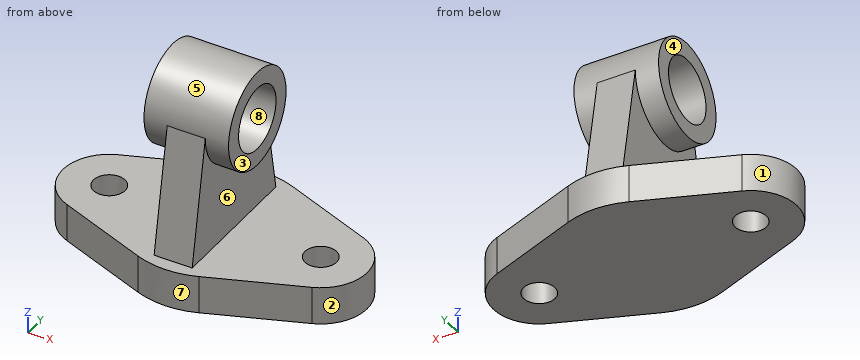
```python
from build123d import *

# Parameters (mm, degrees)
BOSS_EXTRUDE1_DEPTH = 18
SKETCH3_W           = 18
SKETCH3_H           = 67
BOSS_EXTRUDE2_DEPTH = 58
SKETCH4_R           = 23
BOSS_EXTRUDE3_DEPTH = 29
BOSS_EXTRUDE4_START = -40
SKETCH5_R           = 23
BOSS_EXTRUDE4_DEPTH = 40
SKETCH6_R           = 15
CUT_EXTRUDE1_DEPTH  = 141.943250991
CUT_EXTRUDE2_DEPTH  = 135.02238619
SKETCH8_R           = 7.5
CUT_EXTRUDE3_DEPTH  = 116.52056094


with BuildPart() as part:
    # Sketch2 → Boss-Extrude1 (new body)
    with BuildSketch(Plane.XY):
        with BuildLine():
            Line((-57.919997401, 20.524958004), (-14.399995275, 37.31809395))
            ThreePointArc((-14.399995275, 37.31809395), (0, 40), (14.399995275, 37.31809395))
            Line((14.399995275, 37.31809395), (57.919997401, 20.524958004))
            ThreePointArc((57.919997401, 20.524958004), (72, 9.117e-06), (57.920002599, -20.524943336))
            Line((57.920002599, -20.524943336), (14.399995275, -37.31809395))
            ThreePointArc((14.399995275, -37.31809395), (-5.065e-06, -40), (-14.400004725, -37.318090304))
            Line((-14.400004725, -37.318090304), (-57.920002599, -20.524943336))
            ThreePointArc((-57.920002599, -20.524943336), (-72, 9.117e-06), (-57.919997401, 20.524958004))
        make_face()
    extrude(amount=BOSS_EXTRUDE1_DEPTH)

    # Sketch3 → Boss-Extrude2 (add)
    with BuildSketch(Plane.XY.offset(18)):
        Rectangle(SKETCH3_W, SKETCH3_H)
    extrude(amount=BOSS_EXTRUDE2_DEPTH)

    # Sketch4 → Boss-Extrude3 (add)
    with BuildSketch(Plane(origin=(9, 0, 0), x_dir=(0, 0, -1), z_dir=(1, 0, 0))):
        with Locations(Location((-76, 0, 0), (0, 0, 90))):
            Circle(SKETCH4_R)
    extrude(amount=-BOSS_EXTRUDE3_DEPTH)

    # Sketch5 → Boss-Extrude4 (add)
    with BuildSketch(Plane.ZY.offset(20).offset(BOSS_EXTRUDE4_START)):
        with Locations(Location((76, 0, 0), (0, 0, 90))):
            Circle(SKETCH5_R)
    extrude(amount=BOSS_EXTRUDE4_DEPTH)

    # Sketch6 → Cut-Extrude1 (cut, through all)
    with BuildSketch(Plane(origin=(20, 0, 0), x_dir=(0, 0, -1), z_dir=(1, 0, 0))):
        with Locations(Location((-76, 0, 0), (0, 0, 90))):
            Circle(SKETCH6_R)
    extrude(amount=-CUT_EXTRUDE1_DEPTH, mode=Mode.SUBTRACT)

    # Sketch7 → Cut-Extrude2 (cut, through all)
    with BuildSketch(Plane(origin=(9, 0, 0), x_dir=(0, 0, -1), z_dir=(1, 0, 0))):
        Polygon((-18, -33.5), (-76, -23), (-76, -33.5), align=None)
        Polygon((-18, 33.5), (-76, 23), (-76, 33.5), align=None)
    extrude(amount=-CUT_EXTRUDE2_DEPTH, mode=Mode.SUBTRACT)

    # Sketch8 → Cut-Extrude3 (cut, through all)
    with BuildSketch(Plane.XY.offset(18)):
        with Locations((50, 6.331e-06)):
            Circle(SKETCH8_R)
        with Locations((-50, 6.331e-06)):
            Circle(SKETCH8_R)
    extrude(amount=-CUT_EXTRUDE3_DEPTH, mode=Mode.SUBTRACT)


solid = part.part
```
CAD build for the part. Positions are in the model's coordinates, mm. Face numbers are marked on the shaded views. A direction names the side the tool comes from. Round coordinates to 2 decimals unless told otherwise and drop trailing zeros. Loops run counter-clockwise (first coordinate to the right, second up) from the corner with the lowest first, then second, coordinate; pieces in that order, holes last. Notation, with made-up numbers: (0.5, 87) - (7.5, 87) arc R32 cw to (7.5, 114) - close; hole circle Ø1 at (62.5, 6.5). An arc over 180 degrees is marked (long way). Return JSON: item names as keys, results as strings. Group by question number.
Q1. Tool access for the marked faces 1, 2, 3, 4 and 5: list every direction of +Z, -Z, +X, -X, +Y, -Y with a clear straight run to the whole face (end or side of a thin tool).
Q2. Two-plate mould, pull along Y, no slides. Class the marked faces 6, 7 and 8: +Y half, -Y half, draft (parallel to the pull), parting line (faces both ways), or undercut.
Q3. Band-saw the part on A-A on z = 10. Give the cut face in (x, y).
Q4. Flat gauge pins, fed straight in: pin 1 Ø10 at (x, z) = (2, 76.5) entering from -Y; pin 2 Ø3 at (y, z) = (-24, 60) entering from +X; pin 3 Ø14 at (y, z) = (-10.5, 65.5) entering from -X; pin 4 Ø17 at (x, y) = (-50, 0) entering from -Z. Where does each tip first touch, or does it go through?
Q5. Band-saw the part on C-C on x = -50. Give the cut face in (y, z), plus the area to 3 significant figures.
Q6. Drill centre lines: line 1 along X through (y, z) = (14.5, 35); line 2 along Y through (x, z) = (-50, 11); line 3 along Z through (x, y) = (-6.5, -10). Where is each one in solid material? Low to high. Write a range as [from, to].
Q7. Band-saw the part on D-D on y = 28. Give the cut face in (x, z).
Q8. Band-saw the part on B-B on y = 12.5. Give the cut face in (x, z), plus the area to 3 significant figures.
Solutions:
{
 "1": {"face 1": "+Z, -Z, -X", "face 2": "+Z, -Z, +X", "face 3": "+Z, +X, +Y, -Y", "face 4": "+Z, -X, +Y, -Y", "face 5": "none"},
 "2": {"face 6": "draft", "face 7": "-Y half", "face 8": "undercut"},
 "3": {"outline": "(-57.92, -20.52) - (-14.4, -37.32) arc R40 ccw to (14.4, -37.32) - (57.92, -20.52) arc R22 ccw to (57.92, 20.52) - (14.4, 37.32) arc R40 ccw to (-14.4, 37.32) - (-57.92, 20.52) arc R22 ccw to start; hole circle Ø15 at (-50, 0); hole circle Ø15 at (50, 0)"},
 "4": {"pin 1": "stops at y = -23.81", "pin 2": "stops at x = 9", "pin 3": "stops at x = -20", "pin 4": "stops at z = 0"},
 "5": {"outline": "(-23.58, 0) - (-7.5, 0) - (-7.5, 18) - (-23.58, 18) - close; (7.5, 0) - (23.58, 0) - (23.58, 18) - (7.5, 18) - close", "area": "579 mm^2"},
 "6": {"line 1": "x = [-9, 9]", "line 2": "y = [-23.58, -7.5], [7.5, 23.58]", "line 3": "z = [0, 64.82], [87.18, 96.71]"},
 "7": {"outline": "(-38.55, 0) - (38.55, 0) - (38.55, 18) - (9, 18) - (9, 48.38) - (-9, 48.38) - (-9, 18) - (-38.55, 18) - close"},
 "8": {"outline": "(-68.1, 0) - (68.1, 0) - (68.1, 18) - (9, 18) - (9, 56.69) - (20, 56.69) - (20, 67.71) - (-20, 67.71) - (-20, 56.69) - (-9, 56.69) - (-9, 18) - (-68.1, 18) - close; (-20, 84.29) - (20, 84.29) - (20, 95.31) - (-20, 95.31) - close", "area": "4,030 mm^2"}
}
